Here's the drawing with two shaded views (mm, measured from the low corner). I have some questions. A direction names the side the tool comes from. Give positions to 0.01 mm unless a question says otherwise; leave off trailing zeros. Loops run counter-clockwise (first coordinate to the right, second up) from the corner with the lowest first, then second, coordinate; pieces in that order, holes last. Notation, with made-up numbers: (42.25, 68) - (48.25, 68) arc R19 ccw to (48.25, 80) - close; hole circle Ø8 at (65, 10). An arc over 180 degrees is marked (long way). Write each question's results on one line, items separated by ' | '. Start each with the question number.
1) I want a section at D-D, the plane y = 35. Write out the boundary of the cut face in (x, z), and give its area (3 significant figures).
2) I want a section at A-A, the plane z = 23.9. Write out the boundary of the cut face in (x, y), and give its area (3 significant figures).
3) If we mould it in two halves opening along X, with no side actions, what happens to the marked faces 3, 4, 5 and 6? For each: +X half, -X half, draft (parallel to the pull), parting line (faces both ways), or undercut.
4) I want a section at B-B, the plane y = 24. Write out the boundary of the cut face in (x, z).
5) On a 3-axis mill with a long thin cutter (end or side, diameter ignored), from which of +Z, -Z, +X, -X, +Y, -Y can I reach the whole of each face in a straight line? I mean the marked faces 1 and 2. Say none if no direction works.
6) I want a section at C-C, the plane x = 23.9. Write out the boundary of the cut face in (y, z), and give its area (3 significant figures).
7) I'm going to push flat-ended pins straight in: pin 1 (2 mm diameter, centred on x = 8.5, y = 66.5, fed in from -Z) (1 decimal); pin 2 (6 mm diameter, centred on x = 13.5, z = 39, fed in from +Y); pin 3 (10 mm diameter, centred on y = 11.5, z = 6.5, fed in from +X); pin 4 (3 mm diameter, centred on y = 35, z = 23.9, fed in from -X). Where does each tip first touch, or does it pass through?
8) If I drill on probe 1 along Z at (x, y) = (24.5, 73); probe 2 along Y at (x, z) = (6, 23); probe 3 along X at (y, z) = (28, 23), over which ranges is the centre line in solid material (lowest first)? Write a range as [from, to].
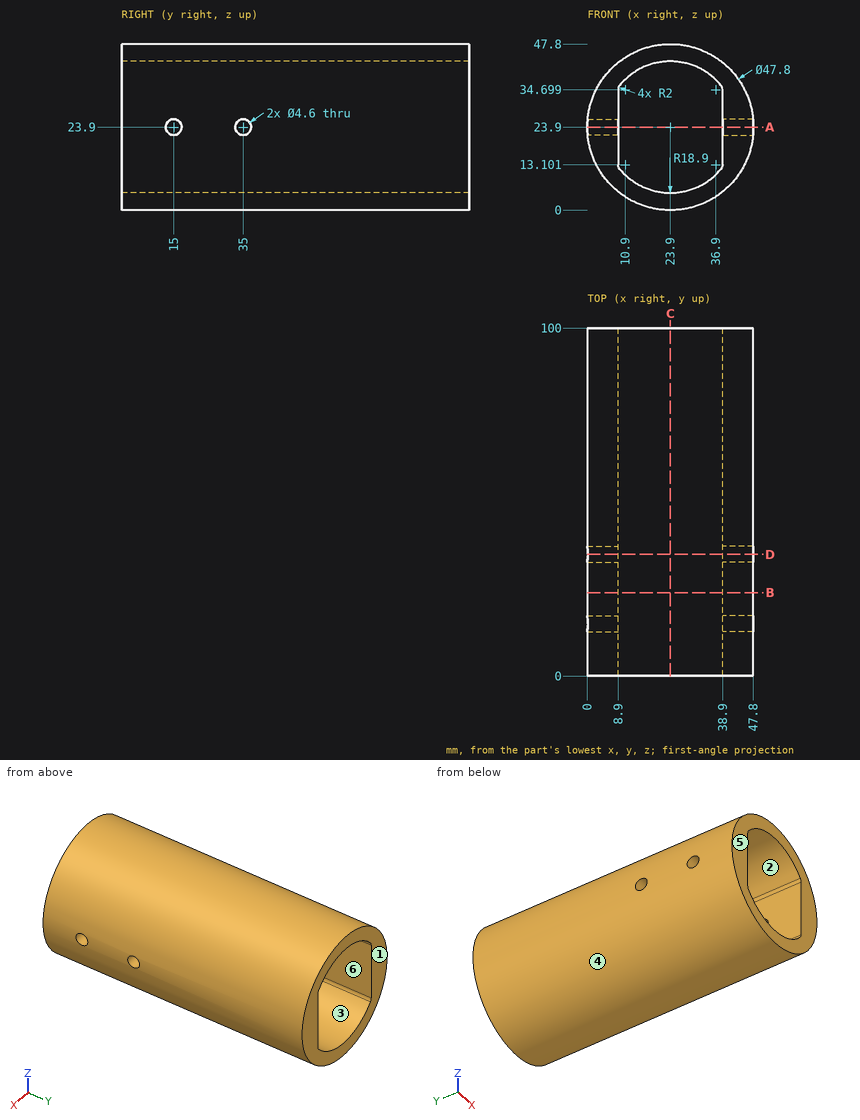
Answers:
1) outline: (0.11, 21.6) arc R23.9 ccw to (47.69, 21.6) - (38.9, 21.6) - (38.9, 13.1) arc R2 cw to (38.44, 11.82) arc R18.9 cw to (9.36, 11.82) arc R2 cw to (8.9, 13.1) - (8.9, 21.6) - close; (0.11, 26.2) - (8.9, 26.2) - (8.9, 34.7) arc R2 cw to (9.36, 35.98) arc R18.9 cw to (38.44, 35.98) arc R2 cw to (38.9, 34.7) - (38.9, 26.2) - (47.69, 26.2) arc R23.9 ccw to start | area: 713 mm2
2) outline: (0, 0) - (8.9, 0) - (8.9, 12.7) - (0, 12.7) - close; (0, 17.3) - (8.9, 17.3) - (8.9, 32.7) - (0, 32.7) - close; (0, 37.3) - (8.9, 37.3) - (8.9, 100) - (0, 100) - close; (38.9, 0) - (47.8, 0) - (47.8, 12.7) - (38.9, 12.7) - close; (38.9, 17.3) - (47.8, 17.3) - (47.8, 32.7) - (38.9, 32.7) - close; (38.9, 37.3) - (47.8, 37.3) - (47.8, 100) - (38.9, 100) - close | area: 1,620 mm2
3) face 3: undercut | face 4: parting line | face 5: draft | face 6: undercut
4) outline: circle Ø47.8 at (23.9, 23.9); hole (8.9, 13.1) arc R2 ccw to (9.36, 11.82) arc R18.9 ccw to (38.44, 11.82) arc R2 ccw to (38.9, 13.1) - (38.9, 34.7) arc R2 ccw to (38.44, 35.98) arc R18.9 ccw to (9.36, 35.98) arc R2 ccw to (8.9, 34.7) - close
5) face 1: +Z, -Z, +X, -X, +Y | face 2: +Y, -Y
6) outline: (0, 0) - (100, 0) - (100, 5) - (0, 5) - close; (0, 42.8) - (100, 42.8) - (100, 47.8) - (0, 47.8) - close | area: 1,000 mm2
7) pin 1: stops at z = 4.8 | pin 2: stops at y = 100 | pin 3: stops at x = 44.33 | pin 4: passes through
8) probe 1: z = [0.01, 5.01], [42.79, 47.79] | probe 2: y = [0, 12.88], [17.12, 32.88], [37.12, 100] | probe 3: x = [0.02, 8.9], [38.9, 47.78]
